Check sheet for the modelled part. Datum: model origin and axes. Units: mm. Face numbers are marked on the shaded views. A direction names the side the tool comes from. Round coordinates to 2 decimals unless told otherwise and drop trailing zeros. Loops run counter-clockwise (first coordinate to the right, second up) from the corner with the lowest first, then second, coordinate; pieces in that order, holes last. Notation, with made-up numbers: M 79,-24 L 103,-24 A34 ccw 103,12 Z; hole C 58.25,27.5 d1. An arc over 180 degrees is marked long. Write item = value, one per line. Start each with the question number.
(1) Mould release check, pull along X, two halves, no side actions. Record for the marked faces 1, 2 and 3: pulls with the +X half, pulls with the -X half, needs draft (parallel to the pull), parting line crosses it, or undercut.
(2) Cross-section at C-C on z = 6.5. Record the boundary of the cut face in (x, y).
(3) Cross-section at B-B on x = -7. Record the boundary of the cut face in (y, z), plus the area to 3 significant figures.
(4) Set-up check for the marked faces 4, 5 and 6: record each of +Z, -Z, +X, -X, +Y, -Y from which the full face is reachable in a straight line by a thin tool's end or side.
(5) Cross-section at A-A on y = 0. Record the boundary of the cut face in (x, z), plus the area to 3 significant figures.
(6) Go/stop test with flat-tipped pins: P1, Ø3, axis at x = -1.5, y = 5.5, coming from the +Z side; P2, Ø2, axis at x = 13, z = 16.5, coming from the +Y side; P3, Ø3, axis at x = 13.5, y = 7.5, coming from the +Z side. Record where each tip stops, or that it passes through.
(7) Scan lines: L1, parallel to Y at x = 0, z = 19.45; L2, parallel to X at y = 7, z = 20; L3, parallel to X at y = -7, z = 21. Record each from-to range of solid material in increasing order. Write a range as from..to.
(8) Cross-section at D-D on y = -15.5. Record the boundary of the cut face in (x, z), plus the area to 3 significant figures.
from build123d import *

# Parameters (mm, degrees)
SKETCH1_R            = 18.4
BOSS_EXTRUDE1_DEPTH  = 21.73
SKETCH2_R            = 17.4
BOSS_EXTRUDE2_DEPTH  = 31
SKETCH3_R            = 6
BOSS_EXTRUDE3_DEPTH  = 6.5
FILLET1_R            = 0.5
SKETCH4_R            = 3
BOSS_EXTRUDE4_DEPTH  = 15.5
CUT_EXTRUDE1_START   = -12
CUT_EXTRUDE1_DEPTH   = 12
CUT_EXTRUDE2_DEPTH   = 1
SKETCH9_R            = 4
BOSS_EXTRUDE5_DEPTH  = 1
FILLET2_R            = 0.5
SKETCH10_R           = 14
BOSS_EXTRUDE6_DEPTH  = 1.5
SKETCH11_W           = 3.5
SKETCH11_H           = 1
BOSS_EXTRUDE7_DEPTH  = 5.6
FILLET3_R            = 0.5
SKETCH13_R           = 9
BOSS_EXTRUDE8_DEPTH  = 3
SKETCH14_R           = 1.5
BOSS_EXTRUDE9_DEPTH  = 8.55
FILLET4_R            = 0.5
SKETCH15_R           = 16.4
BOSS_EXTRUDE10_DEPTH = 15.26
SKETCH17_R           = 1.8
CUT_EXTRUDE3_DEPTH   = 3


with BuildPart() as part:
    # Sketch1 → Boss-Extrude1 (new body)
    with BuildSketch(Plane.XY):
        Circle(SKETCH1_R)
    extrude(amount=BOSS_EXTRUDE1_DEPTH)

    # Sketch2 → Boss-Extrude2 (add)
    with BuildSketch(Plane(origin=(0, 0, 0), x_dir=(-1, 0, 0), z_dir=(0, 0, -1))):
        with Locations(Location((0, 0, 0), (0, 0, 180))):
            Circle(SKETCH2_R)
    extrude(amount=BOSS_EXTRUDE2_DEPTH)

    # Sketch3 → Boss-Extrude3 (add)
    with BuildSketch(Plane.XY.offset(21.73)):
        with Locations(Location((7, 0, 0), (0, 0, 180))):
            Circle(SKETCH3_R)
    extrude(amount=BOSS_EXTRUDE3_DEPTH)

    # Fillet1
    fillet1_edges = [part.edges().sort_by_distance(p)[0] for p in [
        (13, 0, 28.23),
    ]]
    fillet(fillet1_edges, radius=FILLET1_R)

    # Sketch4 → Boss-Extrude4 (add)
    with BuildSketch(Plane.XY.offset(28.23)):
        with Locations((7, 0)):
            Circle(SKETCH4_R)
    extrude(amount=BOSS_EXTRUDE4_DEPTH)

    # Sketch5 → Cut-Extrude1 (cut)
    with BuildSketch(Plane.XY.offset(43.73).offset(CUT_EXTRUDE1_START)):
        with BuildLine():
            Line((5.503337045, 2.6), (8.496662955, 2.6))
            ThreePointArc((8.496662955, 2.6), (7, 3), (5.503337045, 2.6))
        make_face()
    extrude(amount=CUT_EXTRUDE1_DEPTH, mode=Mode.SUBTRACT)

    # Sketch8 → Cut-Extrude2 (cut)
    with BuildSketch(Plane.XY.offset(21.73)):
        with BuildLine():
            ThreePointArc((10.116155685, 7.342574083), (-12.5, 0), (10.116155685, -7.342574083))
            ThreePointArc((10.116155685, -7.342574083), (-1.05978604, 0), (10.116155685, 7.342574083))
        make_face()
    extrude(amount=-CUT_EXTRUDE2_DEPTH, mode=Mode.SUBTRACT)

    # Sketch9 → Boss-Extrude5 (add)
    with BuildSketch(Plane(origin=(0, 0, -31), x_dir=(-1, 0, 0), z_dir=(0, 0, -1))):
        Circle(SKETCH9_R)
    extrude(amount=BOSS_EXTRUDE5_DEPTH)

    # Fillet2
    fillet2_edges = [part.edges().sort_by_distance(p)[0] for p in [
        (4, 0, -32),
    ]]
    fillet(fillet2_edges, radius=FILLET2_R)

    # Sketch11 → Boss-Extrude7 (add)
    with BuildSketch(Plane(origin=(0, 0, -31), x_dir=(-1, 0, 0), z_dir=(0, 0, -1))):
        with Locations((0, 12.05)):
            Rectangle(SKETCH11_W, SKETCH11_H)
        with Locations((0, -12.05)):
            Rectangle(SKETCH11_W, SKETCH11_H)
    extrude(amount=BOSS_EXTRUDE7_DEPTH)

    # Fillet3
    fillet3_edges = [part.edges().sort_by_distance(p)[0] for p in [
        (1.75, 12.05, -36.6),
        (-1.75, 12.05, -36.6),
        (-1.75, -12.05, -36.6),
        (1.75, -12.05, -36.6),
    ]]
    fillet(fillet3_edges, radius=FILLET3_R)

    # Sketch14 → Boss-Extrude9 (add)
    with BuildSketch(Plane(origin=(0, 0, -32), x_dir=(-1, 0, 0), z_dir=(0, 0, -1))):
        Circle(SKETCH14_R)
    extrude(amount=BOSS_EXTRUDE9_DEPTH)

    # Fillet4
    # the kernel refuses this fillet: 0.5 mm, written as the material it takes off along each edge
    with BuildSketch(Plane(origin=(7, 0, 43.73), x_dir=(0.4622655728594592, 0.8867415295050277, 0), z_dir=(0.8867415295050277, -0.4622655728594592, 0))) as fillet4_piece_1:
        with BuildLine():
            CenterArc((3 - FILLET4_R, -FILLET4_R), FILLET4_R, 0, 90)
            Line((3 - FILLET4_R, 0), (3 - FILLET4_R, FILLET4_R * 0.02))
            Line((3 - FILLET4_R, FILLET4_R * 0.02), (3 + FILLET4_R * 0.02, FILLET4_R * 0.02))
            Line((3 + FILLET4_R * 0.02, FILLET4_R * 0.02), (3 + FILLET4_R * 0.02, -FILLET4_R))
            Line((3 + FILLET4_R * 0.02, -FILLET4_R), (3, -FILLET4_R))
        make_face()
    revolve(axis=Axis((7, 0, 43.73), (0, 0, 1)), revolution_arc=297.533397677, mode=Mode.SUBTRACT)
    with BuildSketch(Plane(origin=(7, 0, 43.73), x_dir=(1, 0, 0), z_dir=(0, -1, 0))) as fillet4_piece_2:
        with BuildLine():
            CenterArc((3 - FILLET4_R, -FILLET4_R), FILLET4_R, 0, 90)
            Line((3 - FILLET4_R, 0), (3 - FILLET4_R, FILLET4_R * 0.02))
            Line((3 - FILLET4_R, FILLET4_R * 0.02), (3 + FILLET4_R * 0.02, FILLET4_R * 0.02))
            Line((3 + FILLET4_R * 0.02, FILLET4_R * 0.02), (3 + FILLET4_R * 0.02, -FILLET4_R))
            Line((3 + FILLET4_R * 0.02, -FILLET4_R), (3, -FILLET4_R))
        make_face()
    revolve(axis=Axis((7, 0, 43.73), (0, 0, 1)), revolution_arc=117.379597562, mode=Mode.SUBTRACT)



with BuildPart() as body_2:
    # Sketch10 → Boss-Extrude6 (new body)
    with BuildSketch(Plane(origin=(0, 0, -34), x_dir=(-1, 0, 0), z_dir=(0, 0, -1))):
        Circle(SKETCH10_R)
    extrude(amount=BOSS_EXTRUDE6_DEPTH)


with BuildPart() as body_3:
    # Sketch13 → Boss-Extrude8 (new body)
    with BuildSketch(Plane(origin=(0, 0, -37.5), x_dir=(-1, 0, 0), z_dir=(0, 0, -1))):
        Circle(SKETCH13_R)
    extrude(amount=BOSS_EXTRUDE8_DEPTH)


with BuildPart() as part_1:
    add(part.part)

    add(body_2.part)  # Boss-Extrude10 merges body 2

    add(body_3.part)  # Boss-Extrude10 merges body 3
    # Sketch15 → Boss-Extrude10 (add)
    with BuildSketch(Plane(origin=(0, 0, -31), x_dir=(-1, 0, 0), z_dir=(0, 0, -1))):
        Circle(SKETCH15_R)
    extrude(amount=BOSS_EXTRUDE10_DEPTH)

    # Sketch17 → Cut-Extrude3 (cut)
    with BuildSketch(Plane.XY.offset(21.73)):
        with Locations((0, -15.5)):
            Circle(SKETCH17_R)
        with Locations((-13.423393759, -7.75)):
            Circle(SKETCH17_R)
        with Locations((-13.423393759, 7.75)):
            Circle(SKETCH17_R)
        with Locations((0, 15.5)):
            Circle(SKETCH17_R)
        with Locations((13.423393759, 7.75)):
            Circle(SKETCH17_R)
        with Locations((13.423393759, -7.75)):
            Circle(SKETCH17_R)
    extrude(amount=-CUT_EXTRUDE3_DEPTH, mode=Mode.SUBTRACT)


solid = part_1.part
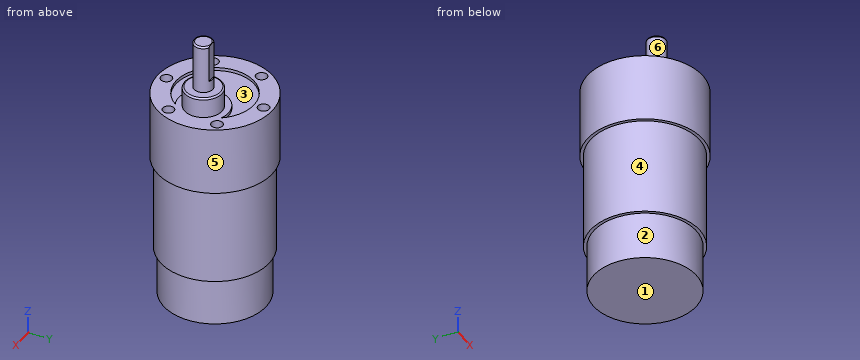
Result:
q1.face_1 = needs draft
q1.face_2 = parting line crosses it
q1.face_3 = undercut
q2.outline = C 0,0 d36.8
q3.outline = M -17.02,0 L -15.93,0 L -15.93,-31 L -14.83,-31 L -14.83,-46.26 L 14.83,-46.26 L 14.83,-31 L 15.93,-31 L 15.93,0 L 17.02,0 L 17.02,21.73 L 10.36,21.73 L 10.36,20.73 L -10.36,20.73 L -10.36,21.73 L -17.02,21.73 Z
q3.area = 2,160 mm^2
q4.face_4 = -Z
q4.face_5 = +Z, -Z
q4.face_6 = +Z
q5.outline = M -18.4,0 L -17.4,0 L -17.4,-31 L -16.4,-31 L -16.4,-46.26 L 16.4,-46.26 L 16.4,-31 L 17.4,-31 L 17.4,0 L 18.4,0 L 18.4,21.73 L 13,21.73 L 13,27.73 A0.5 ccw 12.5,28.23 L 10,28.23 L 10,43.23 A0.5 ccw 9.5,43.73 L 4.5,43.73 A0.5 ccw 4,43.23 L 4,28.23 L 1.5,28.23 A0.5 ccw 1,27.73 L 1,21.73 L -1.06,21.73 L -1.06,20.73 L -12.5,20.73 L -12.5,21.73 L -18.4,21.73 Z
q5.area = 2,540 mm^2
q6.P1 = 20.73
q6.P2 = 13.95
q6.P3 = 18.73
q7.L1 = -18.4..-17.3, -13.7..13.7, 17.3..18.4
q7.L2 = -17.02..-15.06, -11.79..11.79, 15.06..17.02
q7.L3 = -17.02..-15.06, -11.79..-10.36, 3.07..11.79, 15.06..17.02
q8.outline = M -9.92,0 L -7.91,0 L -7.91,-31 L -5.36,-31 L -5.36,-46.26 L 5.36,-46.26 L 5.36,-31 L 7.91,-31 L 7.91,0 L 9.92,0 L 9.92,21.73 L 1.8,21.73 L 1.8,18.73 L -1.8,18.73 L -1.8,21.73 L -9.92,21.73 Z
q8.area = 1,070 mm^2
